Drawing for the job (mm, zero at the part's lowest x, y, z). Give positions to 0.01 mm unless a question says otherwise; leave off trailing zeros. Order: outer loops, then holes, each group sorted by start corner. A loop starts at its lowest first (then second) coordinate and runs counter-clockwise, first axis right, second up. Notation, with made-up numbers: M 67.25,27.25 L 79.25,27.25 A32 cw 79.25,64.25 Z; hole C 19.5,-40 d11. An arc over 180 degrees is marked long. Answer as a JSON object with one key per item and string values.
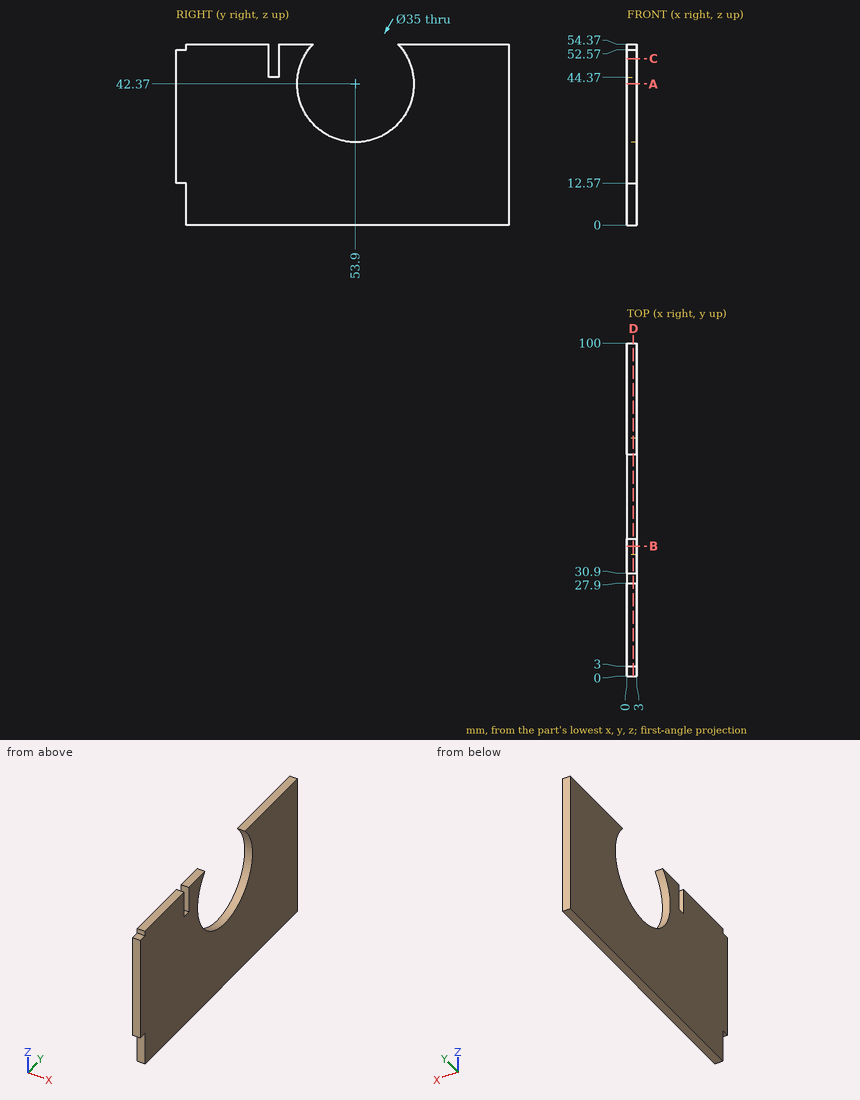
1. Probe line 1 along Y through (x, z) = (0.9, 42.37); line 2 along Z through (x, y) = (1.3, 53.9); line 3 along Y through (x, z) = (2.2, 31). List the from-to ranges inside material, lowest first.
Worked answers:
{"line 1": "y = 0 to 36.4, 71.4 to 100", "line 2": "z = 0 to 24.87", "line 3": "y = 0 to 40.6, 67.2 to 100"}
2. Cut at B-B on y = 39. Give the cut face in (x, z), plus the area to 3 significant figures.
Worked answers:
{"outline": "M 0,0 L 3,0 L 3,33.19 L 0,33.19 Z; M 0,51.55 L 3,51.55 L 3,54.37 L 0,54.37 Z", "area": "108 mm^2"}
3. Cut at C-C on z = 50. Give the cut face in (x, y).
Worked answers:
{"outline": "M 0,0 L 3,0 L 3,27.9 L 0,27.9 Z; M 0,30.9 L 3,30.9 L 3,38.15 L 0,38.15 Z; M 0,69.65 L 3,69.65 L 3,100 L 0,100 Z"}
4. Cut at A-A on z = 42.37. Give the cut face in (x, y), plus the area to 3 significant figures.
Worked answers:
{"outline": "M 0,0 L 3,0 L 3,36.4 L 0,36.4 Z; M 0,71.4 L 3,71.4 L 3,100 L 0,100 Z", "area": "195 mm^2"}
5. Pin check, flat tips, straight feed: P1, Ø1.5, axis at x = 2, y = 1.5, coming from the -Z side; P2, Ø1.4, axis at x = 1.5, z = 54, coming from the -Y side. Stop position of each tip, or through.
Worked answers:
{"P1": "stops at z = 12.57", "P2": "stops at y = 3"}
6. Cut at D-D on x = 1.9. Give the cut face in (y, z).
Worked answers:
{"outline": "M 0,12.57 L 3,12.57 L 3,0 L 100,0 L 100,54.37 L 66.64,54.37 A17.5 cw long 41.16,54.37 L 30.9,54.37 L 30.9,44.37 L 27.9,44.37 L 27.9,54.37 L 3,54.37 L 3,52.57 L 0,52.57 Z"}
